Part model, mm, in its own coordinate system. Coordinates: 2 decimals unless noted, no trailing zeros. Write each loop counter-clockwise with the first axis right and the second up, starting at its lowest first coordinate (ties: lowest second). Pieces come first, ordered by that corner, then holes. Notation, with made-up numbers: (-22.5, 61.25) - (24.5, 61.25) arc R24 cw to (24.5, 77.25) - close; hole circle Ø11 at (65.25, -25.75). An arc over 180 degrees is marked (long way). Use a Markdown table: item, result.
```python
from build123d import *

# Parameters (mm, degrees)
F1_DEPTH = 12.7
F2_R     = 5.08
F3_W     = 402.312346
F3_H     = 25.619045
F4_DEPTH = 73.66
F5_R     = 13.081
F6_DEPTH = 6.35


with BuildPart() as f1:
    # F0 (on Front) → F1 (new body)
    with BuildSketch(Plane.XZ):
        with BuildLine():
            Line((0, 203.2), (0, 0))
            Line((0, 0), (250.542982, 0))
            Line((250.542982, 0), (250.542982, 41.870144))
            Line((250.542982, 41.870144), (188.859552, 122.602507))
            Line((188.859552, 122.602507), (172.564591, 122.602507))
            ThreePointArc((172.564591, 122.602507), (159.229591, 109.267507), (145.894591, 122.602507))
            Line((145.894591, 122.602507), (125.359552, 122.602507))
            Line((125.359552, 122.602507), (63.5, 203.2))
            Line((63.5, 203.2), (45.085, 203.2))
            ThreePointArc((45.085, 203.2), (31.75, 189.865), (18.415, 203.2))
            Line((18.415, 203.2), (0, 203.2))
        make_face()
    extrude(amount=F1_DEPTH)

    # F2
    f2_edges = [f1.edges().sort_by_distance(p)[0] for p in [
        (0, -12.7, 101.6),
        (125.271491, -12.7, 0),
        (250.542982, -12.7, 20.935072),
        (219.701267, -12.7, 82.236326),
        (180.712072, -12.7, 122.602507),
        (159.229591, -12.7, 109.267507),
        (135.627072, -12.7, 122.602507),
        (94.429776, -12.7, 162.901254),
        (54.2925, -12.7, 203.2),
        (31.75, -12.7, 189.865),
        (9.2075, -12.7, 203.2),
        (0, 0, 101.6),
        (125.271491, 0, 0),
        (250.542982, 0, 20.935072),
        (219.701267, 0, 82.236326),
        (180.712072, 0, 122.602507),
        (159.229591, 0, 109.267507),
        (135.627072, 0, 122.602507),
        (94.429776, 0, 162.901254),
        (54.2925, 0, 203.2),
        (31.75, 0, 189.865),
        (9.2075, 0, 203.2),
    ]]
    fillet(f2_edges, radius=F2_R)

    # F3 (on Front) → F4 (cut, symmetric)
    with BuildSketch(Plane.XZ):
        with Locations((92.536684, -6.778551)):
            Rectangle(F3_W, F3_H)
    extrude(amount=F4_DEPTH, both=True, mode=Mode.SUBTRACT)

    # F5 (on Front) → F6 (cut)
    with BuildSketch(Plane.XZ):
        with Locations((62.512301, 62.07348)):
            Circle(F5_R)
    extrude(amount=F6_DEPTH, mode=Mode.SUBTRACT)


solid = f1.part
```
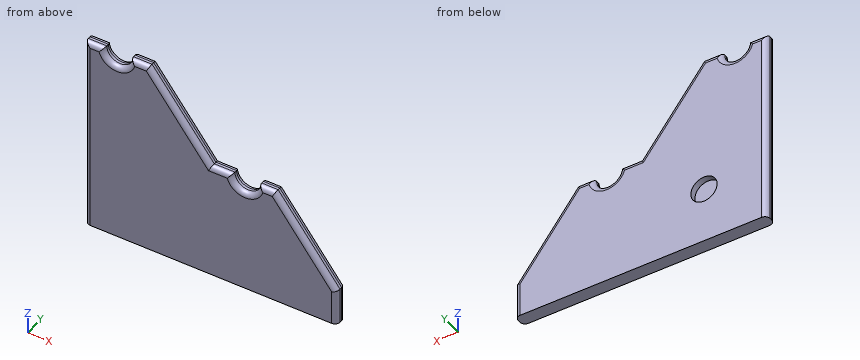
Item 1: Drill centre lines: probe 1 along X at (y, z) = (-4.5, 40); probe 2 along Z at (x, y) = (173.5, -7); probe 3 along X at (y, z) = (-1.25, 193.5). Where is each one in solid material? Low to high.
From the geometry:
| item | result |
|---|---|
| probe 1 | 0.03 to 250.51 |
| probe 2 | 6.03 to 122.6 |
| probe 3 | 1.74 to 20.21, 43.29 to 68.75 |
Item 2: Drop flat-ended pins along their axis: P1, Ø4, axis at y = -2.5, z = 94, coming from the -X side; P2, Ø1.3, axis at x = 135.5, y = -7, coming from the +Z side; P3, Ø21, axis at x = 61.5, z = 55.5, coming from the +Y side. Give the stop position or say it passes through.
From the geometry:
| item | result |
|---|---|
| P1 | x = 0.03 |
| P2 | z = 122.6 |
| P3 | y = 0 |
Item 3: Band-saw the part on A-A, the plane x = 31.75. Give the cut face in (y, z) (3 decimals).
From the geometry:
| item | result |
|---|---|
| outline | (-12.7, 6.031) - (0, 6.031) - (0, 184.785) arc R5.08 ccw to (-5.08, 189.865) - (-7.62, 189.865) arc R5.08 ccw to (-12.7, 184.785) - close |
Item 4: Band-saw the part on B-B, the plane x = 138. Give the cut face in (y, z).
From the geometry:
| item | result |
|---|---|
| outline | (-12.7, 6.03) - (0, 6.03) - (0, 117.52) arc R5.08 ccw to (-5.08, 122.6) - (-7.62, 122.6) arc R5.08 ccw to (-12.7, 117.52) - close |
